Build history of the part. All positions in model axes, mm. Coordinates: 2 decimals unless noted, no trailing zeros. Loops run counter-clockwise (first coordinate to the right, second up) from the corner with the lowest first, then second, coordinate; pieces in that order, holes last. Notation, with made-up numbers: (70, -24.5) - (81, -24.5) arc R12 ccw to (81, -15.5) - close; hole circle Ø4 at (-2.5, 48). An arc over 180 degrees is marked (long way). One line per item, written item: value.
```python
from build123d import *

# Parameters (mm, degrees)
F0_W     = 100
F0_H     = 100
F1_DEPTH = 16.5
F2_R     = 0.25
F3_DEPTH = 16.501
F4_R     = 35
F4_R_2   = 0.25
F5_DEPTH = 6.5


with BuildPart() as f1:
    # F0 (on Front) → F1 (new body)
    with BuildSketch(Plane.XZ):
        Rectangle(F0_W, F0_H)
    extrude(amount=F1_DEPTH)

    # F2 (on face) → F3 (cut, through all)
    with BuildSketch(Plane.XZ.offset(16.5)):
        Circle(F2_R)
    extrude(amount=-F3_DEPTH, mode=Mode.SUBTRACT)

    # F4 (on face) → F5 (cut)
    with BuildSketch(Plane(origin=(0, 0, 0), x_dir=(-1, 0, 0), z_dir=(0, 1, 0))):
        Circle(F4_R)
        Circle(F4_R_2, mode=Mode.SUBTRACT)
    extrude(amount=-F5_DEPTH, mode=Mode.SUBTRACT)


solid = f1.part
```
Item 1: Cut at C-C, the plane z = 13. Write the cut outline in (x, y).
Check result:
outline: (-50, -16.5) - (50, -16.5) - (50, 0) - (32.5, 0) - (32.5, -6.5) - (-32.5, -6.5) - (-32.5, 0) - (-50, 0) - close
Item 2: Cut at B-B, the plane x = 15. Write the cut outline in (y, z).
Check result:
outline: (-16.5, -50) - (0, -50) - (0, -31.62) - (-6.5, -31.62) - (-6.5, 31.62) - (0, 31.62) - (0, 50) - (-16.5, 50) - close
Item 3: Probe probe 1 along Z at (x, y) = (0, -4.25); probe 2 along X at (y, z) = (-10, 0). List the from-to ranges inside material, lowest first. Write a range as from..to.
Check result:
probe 1: z = -50..-35, 35..50
probe 2: x = -50..-0.25, 0.25..50
Item 4: Pull direction Z, two halves, no side cores. Call faces 1 (the face through (0.5, -6.5, 0.5)), 2 (the face through (28, -3, -21)), 3 (the face through (-1, -8, -50)), 4 (the face through (50, -8, -1)): released by +Z, released by -Z, zero draft, split by the parting line, or undercut.
Check result:
face 1: undercut
face 2: undercut
face 3: released by -Z
face 4: zero draft
Item 5: Cut at A-A, the plane y = -4.75. Write the cut outline in (x, z), then the cut area to 3 significant figures.
Check result:
outline: (-50, -50) - (50, -50) - (50, 50) - (-50, 50) - close; hole circle Ø70 at (0, 0)
area: 6,150 mm^2
Item 6: Drop a flat-ended pin along its axis: P1, Ø6, axis at x = 25, z = -4.5, coming from the +Y side. Give the stop position or say it passes through.
Check result:
P1: stops at y = -6.5
